from build123d import *

# Parameters (mm, degrees)
BASE_SKETCH_W                              = 804.8625
BASE_SKETCH_H                              = 387.35
BASE_SKETCH_R                              = 5.08
BASE_W_MOUNT_HOLES_DEPTH                   = 0.7366
THROTTLE_AND_CHOKE_CUTOUT_SKETCH_R         = 8.89
THROTTLE_AND_CHOKE_CUTOUT_SKETCH_R_2       = 4.318
THROTTLE_AND_CHOKE_CUTOUTS_DEPTH           = 1.7366
STARTER_RELAY_MOUNT_SKETCH_R               = 2.38125
STARTER_RELAY_MOUNT_DEPTH                  = 1.7366
OIL_PRESSURE_SENDER_CLAMP_MOUNT_SKETCH_R   = 2.54
OIL_PRESSURE_SENDER_CLAMP_MOUNT_DEPTH      = 1.7366
STARTER_POWER_CUTOUT_SKETCH_R              = 5.588
STARTER_POWER_CUTOUT_DEPTH                 = 1.7366
FUEL_RETURN_CUTOUT_SKETCH_R                = 7.62
FUEL_RETURN_CUTOUT_DEPTH                   = 1.7366
BRAKE_MASTER_CYL_MOUNT_SKETCH_R            = 1.6256
BRAKE_MASTER_CYL_MOUNT_DEPTH               = 1.7366
CUTOUT_AS012_INSTRUMENTATION_RIGHT_S_R     = 10.94994
CUTOUT_AS012_INSTRUMENTATION_RIGHT_S_R_2   = 1.8034
CUTOUT_AS012_INSTRUMENTATION_RIGHT_DEPTH   = 1.7366
CUTOUT_AS014_TACH_AND_CDI_ENABLE_2_R       = 12.4968
CUTOUT_AS014_TACH_AND_CDI_ENABLE_2_R_2     = 1.8034
CUTOUT_AS014_TACH_AND_CDI_ENABLES_LE_DEPTH = 1.7366
CUTOUT_AS012_INSTRUMENTATION_LEFT_SK_R     = 10.94994
CUTOUT_AS012_INSTRUMENTATION_LEFT_SK_R_2   = 1.6002
CUTOUT_AS012_INSTRUMENTATION_LEFT_DEPTH    = 1.7366


with BuildPart() as part:
    # Base Sketch → Base w Mount Holes (new body)
    with BuildSketch(Plane.XY):
        with Locations((375.44375, 168.275)):
            Rectangle(BASE_SKETCH_W, BASE_SKETCH_H)
        Circle(BASE_SKETCH_R, mode=Mode.SUBTRACT)
        with Locations((750.8875, 0)):
            Circle(BASE_SKETCH_R, mode=Mode.SUBTRACT)
        with Locations((207.565625, 236.5375)):
            Circle(BASE_SKETCH_R, mode=Mode.SUBTRACT)
        with Locations((543.321875, 236.5375)):
            Circle(BASE_SKETCH_R, mode=Mode.SUBTRACT)
    extrude(amount=BASE_W_MOUNT_HOLES_DEPTH)

    # Throttle and Choke Cutout Sketch → Throttle and Choke Cutouts (cut, through all)
    with BuildSketch(Plane.XY.offset(0.7366)):
        with Locations((63.5, 138.1125)):
            Circle(THROTTLE_AND_CHOKE_CUTOUT_SKETCH_R)
        with Locations((63.5, 199.0725)):
            Circle(THROTTLE_AND_CHOKE_CUTOUT_SKETCH_R_2)
        with Locations((687.3875, 199.0725)):
            Circle(THROTTLE_AND_CHOKE_CUTOUT_SKETCH_R_2)
        with Locations((687.3875, 138.1125)):
            Circle(THROTTLE_AND_CHOKE_CUTOUT_SKETCH_R)
    extrude(amount=-THROTTLE_AND_CHOKE_CUTOUTS_DEPTH, mode=Mode.SUBTRACT)

    # Starter Relay Mount Sketch → Starter Relay Mount (cut, through all)
    with BuildSketch(Plane.XY.offset(0.7366)):
        with Locations((149.225, 161.925)):
            Circle(STARTER_RELAY_MOUNT_SKETCH_R)
        with Locations((212.217, 161.925)):
            Circle(STARTER_RELAY_MOUNT_SKETCH_R)
    extrude(amount=-STARTER_RELAY_MOUNT_DEPTH, mode=Mode.SUBTRACT)

    # Oil Pressure Sender Clamp Mount Sketch → Oil Pressure Sender Clamp Mount (cut, through all)
    with BuildSketch(Plane.XY.offset(0.7366)):
        with Locations((76.2, 44.45)):
            Circle(OIL_PRESSURE_SENDER_CLAMP_MOUNT_SKETCH_R)
    extrude(amount=-OIL_PRESSURE_SENDER_CLAMP_MOUNT_DEPTH, mode=Mode.SUBTRACT)

    # Starter Power Cutout Sketch → Starter Power Cutout (cut, through all)
    with BuildSketch(Plane.XY.offset(0.7366)):
        with Locations((233.3625, 33.3375)):
            Circle(STARTER_POWER_CUTOUT_SKETCH_R)
    extrude(amount=-STARTER_POWER_CUTOUT_DEPTH, mode=Mode.SUBTRACT)

    # Fuel Return Cutout Sketch → Fuel Return Cutout (cut, through all)
    with BuildSketch(Plane.XY.offset(0.7366)):
        with Locations((101.6, 104.775)):
            Circle(FUEL_RETURN_CUTOUT_SKETCH_R)
    extrude(amount=-FUEL_RETURN_CUTOUT_DEPTH, mode=Mode.SUBTRACT)

    # Brake Master Cyl Mount Sketch → Brake Master Cyl Mount (cut, through all)
    with BuildSketch(Plane.XY.offset(0.7366)):
        with Locations((546.1, 123.825)):
            Circle(BRAKE_MASTER_CYL_MOUNT_SKETCH_R)
        with Locations((604.52, 123.825)):
            Circle(BRAKE_MASTER_CYL_MOUNT_SKETCH_R)
    extrude(amount=-BRAKE_MASTER_CYL_MOUNT_DEPTH, mode=Mode.SUBTRACT)

    # Cutout - AS012 - Instrumentation Right Sketch → Cutout - AS012 - Instrumentation Right (cut, through all)
    with BuildSketch(Plane.XY.offset(0.7366)):
        with Locations((141.2875, 236.5375)):
            Circle(CUTOUT_AS012_INSTRUMENTATION_RIGHT_S_R)
        with Locations((141.2875, 221.98711)):
            Circle(CUTOUT_AS012_INSTRUMENTATION_RIGHT_S_R_2)
        with Locations((141.2875, 251.08789)):
            Circle(CUTOUT_AS012_INSTRUMENTATION_RIGHT_S_R_2)
    extrude(amount=-CUTOUT_AS012_INSTRUMENTATION_RIGHT_DEPTH, mode=Mode.SUBTRACT)

    # Cutout - AS014 - Tach and CDI Enable 2 → Cutout - AS014 - Tach and CDI Enables Le (cut, through all)
    with BuildSketch(Plane.XY.offset(0.7366)):
        with Locations((609.6, 236.5375)):
            Circle(CUTOUT_AS014_TACH_AND_CDI_ENABLE_2_R)
        with Locations((609.6, 252.78715)):
            Circle(CUTOUT_AS014_TACH_AND_CDI_ENABLE_2_R_2)
        with Locations((609.6, 220.28785)):
            Circle(CUTOUT_AS014_TACH_AND_CDI_ENABLE_2_R_2)
    extrude(amount=-CUTOUT_AS014_TACH_AND_CDI_ENABLES_LE_DEPTH, mode=Mode.SUBTRACT)

    # Cutout - AS012 - Instrumentation Left Sketch → Cutout - AS012 - Instrumentation Left (cut, through all)
    with BuildSketch(Plane.XY.offset(0.7366)):
        with Locations((647.7, 215.9)):
            Circle(CUTOUT_AS012_INSTRUMENTATION_LEFT_SK_R)
        with Locations((647.7, 230.45039)):
            Circle(CUTOUT_AS012_INSTRUMENTATION_LEFT_SK_R_2)
        with Locations((647.7, 201.34961)):
            Circle(CUTOUT_AS012_INSTRUMENTATION_LEFT_SK_R_2)
    extrude(amount=-CUTOUT_AS012_INSTRUMENTATION_LEFT_DEPTH, mode=Mode.SUBTRACT)


solid = part.part
Input: part model. Units: mm. Frame: model coordinates. Coordinates: 2 decimals unless noted, no trailing zeros. Loops run counter-clockwise (first coordinate to the right, second up) from the corner with the lowest first, then second, coordinate; pieces in that order, holes last.
Q1. Draft query along Y for faces 1 (the face through (93.987, 105.11, 0.373)), 2 (the face through (370, 171, 0.737)). Return one class per face: +Y half, -Y half, draft (parallel to the pull), parting line (faces both ways), or undercut.
Q2. Cut plane A-A (x = 101.6). Output: boundary loops of the cut face in (y, z) (3 decimals).
Q3. Material intervals for line 1 (Y direction, x = 609.6, z = 0.2); line 2 (Y direction, x = 647.7, z = 0.5); line 3 (Y direction, x = 76.2, z = 0.3), sorted ascending.
Q4. Contact query for a flat-ended pin moving along its axis: pin 1 (11.5 mm diameter, centred on x = 543.32, y = 236.54, fed in from -Z). Output: stop coordinate, or through.
Working result:
1. face 1: undercut
1. face 2: draft
2. outline: (-25.4, 0) - (97.155, 0) - (97.155, 0.737) - (-25.4, 0.737) - close; (112.395, 0) - (361.95, 0) - (361.95, 0.737) - (112.395, 0.737) - close
3. line 1: y = -25.4 to 218.48, 222.09 to 224.04, 249.03 to 250.98, 254.59 to 361.95
3. line 2: y = -25.4 to 199.75, 202.95 to 204.95, 226.85 to 228.85, 232.05 to 361.95
3. line 3: y = -25.4 to 41.91, 46.99 to 361.95
4. pin 1: stops at z = 0
